Answer from the drawing. Dimensions are ordinates in mm from the lowest x, y and z of the part. A direction names the side the tool comes from. Coordinates: 2 decimals unless noted, no trailing zeros. Write each loop counter-clockwise with the first axis right and the second up, starting at its lowest first coordinate (ties: lowest second). Pieces come first, ordered by that corner, then holes.
(1) The part is cut by section A-A on z = 10.5. Determine the outline of the cut face in (x, y).
(2) Straight lines are drawn through the part: line 1 (X direction, y = 2.3, z = 10.5); line 2 (Y direction, x = 13, z = 1.95); line 3 (Y direction, x = 7, z = 12.25). For each, find the intervals that lie inside material, in ascending order.
(3) The part is cut by section B-B on x = 13. Determine the outline of the cut face in (y, z).
(4) The part is cut by section C-C on y = 3. Determine the outline of the cut face in (x, z), plus the area to 3 significant figures.
(5) For a pull along Z with two mould halves and no side action, classify the marked faces 3, 4 and 5 as +Z half, -Z half, draft (parallel to the pull), parting line (faces both ways), or undercut.
(6) Which of the six approach directions +Z, -Z, +X, -X, +Y, -Y give full straight-line access (tool end or side, diameter ignored) to the marked faces 1 and 2?
(7) Given P1, Ø3, axis at x = 13, z = 10.5, coming from the -Y side; P2, Ø4, axis at y = 29.5, z = 4, coming from the +X side; P3, Ø4.5, axis at x = 17.5, z = 12, coming from the +Y side; P4, Ø3, axis at x = 5.93, y = 12.93, coming from the +Z side, each flat-ended and moving along its own axis, determine where each tip first touches the part or whether it passes through.
(8) The part is cut by section D-D on x = 8.75. Determine the outline of the cut face in (y, z).
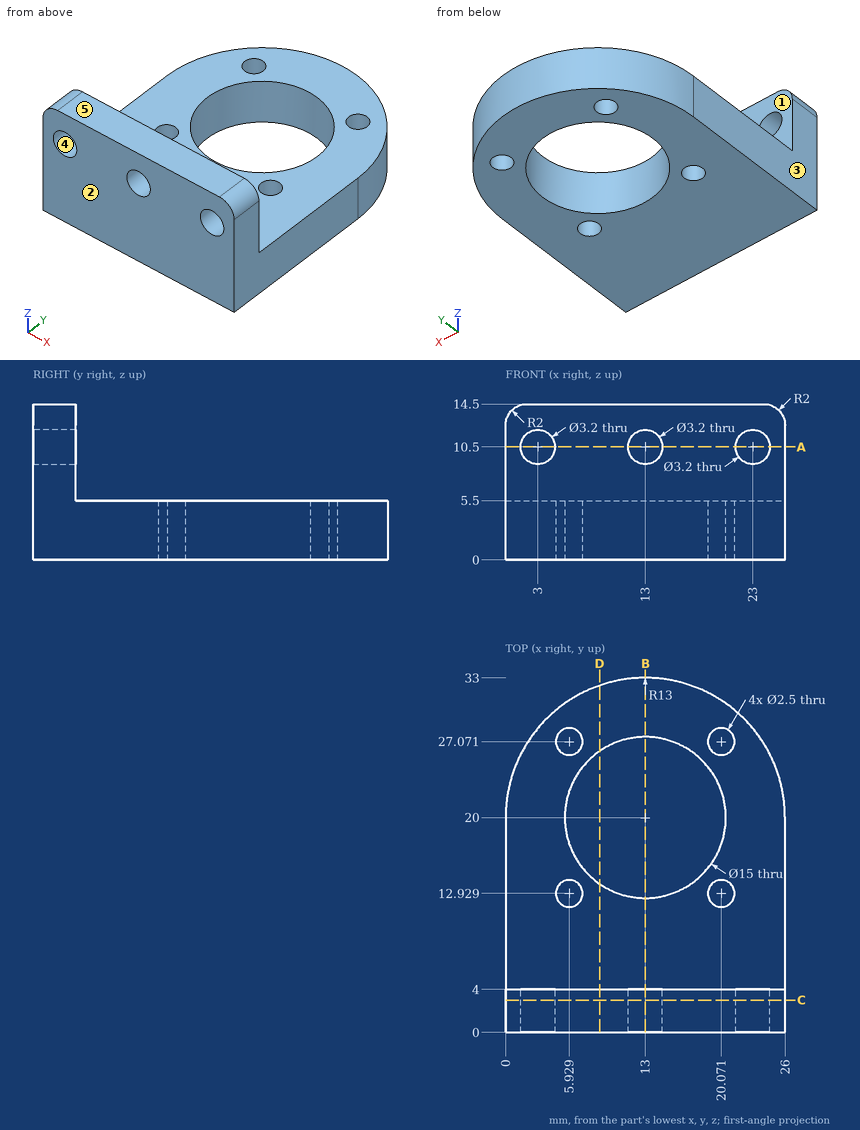
Model answer:
1. outline: (0, 0) - (1.4, 0) - (1.4, 4) - (0, 4) - close; (4.6, 0) - (11.4, 0) - (11.4, 4) - (4.6, 4) - close; (14.6, 0) - (21.4, 0) - (21.4, 4) - (14.6, 4) - close; (24.6, 0) - (26, 0) - (26, 4) - (24.6, 4) - close
2. line 1: x = 0 to 1.4, 4.6 to 11.4, 14.6 to 21.4, 24.6 to 26
2. line 2: y = 0 to 12.5, 27.5 to 33
2. line 3: y = 0 to 4
3. outline: (0, 0) - (12.5, 0) - (12.5, 5.5) - (4, 5.5) - (4, 8.9) - (0, 8.9) - close; (0, 12.1) - (4, 12.1) - (4, 14.5) - (0, 14.5) - close; (27.5, 0) - (33, 0) - (33, 5.5) - (27.5, 5.5) - close
4. outline: (0, 0) - (26, 0) - (26, 12.5) arc R2 ccw to (24, 14.5) - (2, 14.5) arc R2 ccw to (0, 12.5) - close; hole circle Ø3.2 at (3, 10.5); hole circle Ø3.2 at (13, 10.5); hole circle Ø3.2 at (23, 10.5)
4. area: 351 mm2
5. face 3: draft
5. face 4: undercut
5. face 5: +Z half
6. face 1: +Z, +X, -X, +Y
6. face 2: +Z, -Z, +X, -X, -Y
7. P1: passes through
7. P2: stops at x = 23.62
7. P3: stops at y = 4
7. P4: stops at z = 5.5
8. outline: (0, 0) - (13.82, 0) - (13.82, 5.5) - (4, 5.5) - (4, 14.5) - (0, 14.5) - close; (26.18, 0) - (32.29, 0) - (32.29, 5.5) - (26.18, 5.5) - close
